from build123d import *

# Parameters (mm, degrees)
SKETCH1_W               = 47.4
SKETCH1_H               = 8
BOSS_EXTRUDE1_DEPTH     = 9
CUT_EXTRUDE1_DEPTH      = 17
CUT_EXTRUDE1_DEPTH_BACK = 58
SKETCH2_W               = 5
SKETCH2_H               = 3
M2X0_4_TAPPED_HOLE1_D   = 1.6


with BuildPart() as part:
    # Sketch1 → Boss-Extrude1 (new body)
    with BuildSketch(Plane(origin=(0, 0, 0), x_dir=(1, 0, 0), z_dir=(0, 1, 0))):
        with Locations((9.069133192, 9.478435518)):
            Rectangle(SKETCH1_W, SKETCH1_H)
    extrude(amount=BOSS_EXTRUDE1_DEPTH)

    # Sketch2 → Cut-Extrude1 (cut, two sides: drawn at the far end of the back side and taken through both)
    with BuildSketch(Plane(origin=(32.769133192, 0, 0), x_dir=(0, 0, -1), z_dir=(1, 0, 0)).offset(-CUT_EXTRUDE1_DEPTH_BACK)):
        with Locations((7.978435518, 4.5)):
            Rectangle(SKETCH2_W, SKETCH2_H)
    extrude(amount=CUT_EXTRUDE1_DEPTH + CUT_EXTRUDE1_DEPTH_BACK, mode=Mode.SUBTRACT)

    # M2x0.4 Tapped Hole1 (through all)
    with Locations(Plane(origin=(0, 9, 0), x_dir=(1, 0, 0), z_dir=(0, 1, 0))):
        with Locations((-2.780866808, 9.478435518), (20.919133192, 9.478435518)):
            Hole(M2X0_4_TAPPED_HOLE1_D / 2)


solid = part.part
Source: CAD feature listing. Evaluate the final solid. Frame: model axes, mm. A direction names the side the tool comes from. Round coordinates to 2 decimals unless told otherwise and drop trailing zeros. Loops run counter-clockwise (first coordinate to the right, second up) from the corner with the lowest first, then second, coordinate; pieces in that order, holes last.
Q1. Mould query, pull axis X, two halves, no side actions, for faces 3 (the face through (9, 7, -5.478)), 4 (the face through (32.769, 4, -11)), 5 (the face through (-2.6, 1.5, -8.7)). Classes: pulls with the +X half, pulls with the -X half, needs draft (parallel to the pull), parting line crosses it, or undercut.
Q2. Access query for faces 1 (the face through (9, 3, -8)), 2 (the face through (9, 9, -10)). Directions: +Z, -Z, +X, -X, +Y, -Y. A direction counts if a zero-diameter tool reaches every point of the face in a straight line with its end or side. Return the directions, or none.
Q3. Section B-B, the plane x = -8.5. Return loops of the section in (y, z), plus the area to 3 significant figures.
Q4. First-contact query: P1, Ø1.4, axis at x = 20.92, z = -9.48, coming from the -Y side. Flat tip, straight axial feed; report the tip coordinate or a pass-through.
Q5. Section C-C, the plane y = 4.75. Return loops of the section in (x, z), plus the area to 3 significant figures.
Q6. Ray query, line 1 (Y direction, x = 28, z = -7); line 2 (Z direction, x = 29.5, y = 5.25); line 3 (Z direction, x = -2.5, y = 2.5). Return the intervals inside material, ascending.
Q7. Section A-A, the plane z = -7.5. Return loops of the section in (x, y), plus the area to 3 significant figures.
Solutions:
1. face 3: needs draft
1. face 4: pulls with the +X half
1. face 5: undercut
2. face 1: +Z, +X, -X
2. face 2: +Z, -Z, +X, -X, +Y
3. outline: (0, -13.48) - (9, -13.48) - (9, -5.48) - (6, -5.48) - (6, -10.48) - (3, -10.48) - (3, -5.48) - (0, -5.48) - close
3. area: 57.0 mm2
4. P1: passes through
5. outline: (-14.63, -13.48) - (32.77, -13.48) - (32.77, -10.48) - (-14.63, -10.48) - close
5. area: 142 mm2
6. line 1: y = 0 to 3, 6 to 9
6. line 2: z = -13.48 to -10.48
6. line 3: z = -13.48 to -10.23, -8.73 to -5.48
7. outline: (-14.63, 0) - (32.77, 0) - (32.77, 3) - (-14.63, 3) - close; (-14.63, 6) - (32.77, 6) - (32.77, 9) - (-14.63, 9) - close
7. area: 284 mm2
